```python
from build123d import *

# Parameters (mm, degrees)
SKETCH021_W     = 28
SKETCH021_H     = 45
SKETCH021_R     = 1.5
PAD010_DEPTH    = 6
SKETCH022_W     = 7
SKETCH022_H     = 45
SKETCH022_R     = 1.5
SKETCH022_W_2   = 6
SKETCH022_H_2   = 10
SKETCH022_H_3   = 6
PAD011_DEPTH    = 8
SKETCH032_R     = 3.5
POCKET010_DEPTH = 3
POCKET011_DEPTH = 27
SKETCH034_R     = 1.5
POCKET012_DEPTH = 19
SKETCH035_R     = 5
PAD012_DEPTH    = 11
SKETCH036_R     = 5
PAD013_DEPTH    = 11
SKETCH037_R     = 1.5
POCKET013_DEPTH = 20
SKETCH038_R     = 1.5
POCKET014_DEPTH = 20
CHAMFER005_SIZE = 2
CHAMFER006_SIZE = 2
CHAMFER007_SIZE = 2
SKETCH039_W     = 9
SKETCH039_H     = 2
PAD014_DEPTH    = 8
SKETCH040_W     = 8
SKETCH040_H     = 2
PAD015_DEPTH    = 8
CHAMFER008_SIZE = 6
SKETCH041_W     = 6
SKETCH041_H     = 2.3
POCKET015_DEPTH = 6
CHAMFER012_SIZE = 2
PAD017_DEPTH    = 1
SKETCH047_W     = 2.3
SKETCH047_H     = 6
POCKET018_DEPTH = 9


with BuildPart() as part:
    # Sketch021 → Pad010 (new body)
    with BuildSketch(Plane.XZ):
        with Locations((14, 22.5)):
            Rectangle(SKETCH021_W, SKETCH021_H)
        with Locations((4, 32.5)):
            Circle(SKETCH021_R, mode=Mode.SUBTRACT)
        with Locations((24, 32.5)):
            Circle(SKETCH021_R, mode=Mode.SUBTRACT)
        with Locations((4, 12.5)):
            Circle(SKETCH021_R, mode=Mode.SUBTRACT)
        with Locations((24, 12.5)):
            Circle(SKETCH021_R, mode=Mode.SUBTRACT)
    extrude(amount=PAD010_DEPTH)

    # Sketch022 (on Face9 of Pad010) → Pad011 (join)
    with BuildSketch(Plane(origin=(0, 0, 0), x_dir=(1, 0, 0), z_dir=(0, 1, 0))):
        with Locations((3.5, -22.5)):
            Rectangle(SKETCH022_W, SKETCH022_H)
        with Locations((4, -12.5)):
            Circle(SKETCH022_R, mode=Mode.SUBTRACT)
        with Locations((4, -32.5)):
            Circle(SKETCH022_R, mode=Mode.SUBTRACT)
        with Locations((24.5, -22.5)):
            Rectangle(SKETCH022_W, SKETCH022_H)
        with Locations((24, -12.5)):
            Circle(SKETCH022_R, mode=Mode.SUBTRACT)
        with Locations((24, -32.5)):
            Circle(SKETCH022_R, mode=Mode.SUBTRACT)
        with Locations((15.5, -5)):
            Rectangle(SKETCH022_W_2, SKETCH022_H_2)
        with Locations((15.5, -15)):
            Rectangle(SKETCH022_W_2, SKETCH022_H_3)
    extrude(amount=PAD011_DEPTH)

    # Sketch032 → Pocket010 (cut)
    with BuildSketch(Plane(origin=(0, 8, 0), x_dir=(1, 0, 0), z_dir=(0, 1, 0))):
        with Locations((4, -12.5)):
            Circle(SKETCH032_R)
        with Locations((4, -32.5)):
            Circle(SKETCH032_R)
        with Locations((24, -32.5)):
            Circle(SKETCH032_R)
        with Locations((24, -12.5)):
            Circle(SKETCH032_R)
    extrude(amount=-POCKET010_DEPTH, mode=Mode.SUBTRACT)

    # Sketch033 (on Face4 of Pocket010) → Pocket011 (cut)
    with BuildSketch(Plane(origin=(0, 0, 45), x_dir=(-1, 0, 0), z_dir=(0, 0, 1))):
        Polygon((-22, 6), (-8, 6), (-10, 0), (-21, 0), align=None)
    extrude(amount=-POCKET011_DEPTH, mode=Mode.SUBTRACT)

    # Sketch034 (on Face5 of Pocket011) → Pocket012 (cut)
    with BuildSketch(Plane(origin=(0, 0, 18), x_dir=(-1, 0, 0), z_dir=(0, 0, 1))):
        with Locations((-15.5, 3)):
            Circle(SKETCH034_R)
    extrude(amount=-POCKET012_DEPTH, mode=Mode.SUBTRACT)

    # Sketch035 (on Face14 of Pocket012) → Pad012 (join)
    with BuildSketch(Plane(origin=(0, 0, 0), x_dir=(0, 0, -1), z_dir=(-1, 0, 0))):
        with Locations((-5, -3)):
            Circle(SKETCH035_R)
    extrude(amount=PAD012_DEPTH)

    # Sketch036 (on Face21 of Pocket012) → Pad013 (join)
    with BuildSketch(Plane(origin=(28, 0, 0), x_dir=(0, 0, 1), z_dir=(1, 0, 0))):
        with Locations((5, -3)):
            Circle(SKETCH036_R)
    extrude(amount=PAD013_DEPTH)

    # Sketch037 (on Face35 of Pad013) → Pocket013 (cut)
    with BuildSketch(Plane(origin=(-11, 0, 0), x_dir=(0, 0, -1), z_dir=(-1, 0, 0))):
        with Locations((-5, -3)):
            Circle(SKETCH037_R)
    extrude(amount=-POCKET013_DEPTH, mode=Mode.SUBTRACT)

    # Sketch038 (on Face52 of Pocket013) → Pocket014 (cut)
    with BuildSketch(Plane(origin=(39, 0, 0), x_dir=(0, 0, 1), z_dir=(1, 0, 0))):
        with Locations((5, -3)):
            Circle(SKETCH038_R)
    extrude(amount=-POCKET014_DEPTH, mode=Mode.SUBTRACT)

    # Chamfer005
    chamfer005_edges = [part.edges().sort_by_distance(p)[0] for p in [
        (39, 3, 0),
        (-11, 3, 10),
    ]]
    chamfer(chamfer005_edges, length=CHAMFER005_SIZE)

    # Chamfer006
    chamfer006_edges = [part.edges().sort_by_distance(p)[0] for p in [
        (37, 3, 0),
        (-9, 3, 10),
    ]]
    chamfer(chamfer006_edges, length=CHAMFER006_SIZE)

    # Chamfer007
    chamfer007_edges = [part.edges().sort_by_distance(p)[0] for p in [
        (35, 3, 2.2e-05),
        (-7, 3, 9.999978),
    ]]
    chamfer(chamfer007_edges, length=CHAMFER007_SIZE)

    # Sketch039 (on Face4 of Chamfer007) → Pad014 (join)
    with BuildSketch(Plane(origin=(0, 0, 0), x_dir=(0, 0, -1), z_dir=(-1, 0, 0))):
        with Locations((-12.5, -3)):
            Rectangle(SKETCH039_W, SKETCH039_H)
    extrude(amount=PAD014_DEPTH)

    # Sketch040 (on Face48 of Pad014) → Pad015 (join)
    with BuildSketch(Plane(origin=(28, 0, 0), x_dir=(0, 0, 1), z_dir=(1, 0, 0))):
        with Locations((12, -3)):
            Rectangle(SKETCH040_W, SKETCH040_H)
    extrude(amount=PAD015_DEPTH)

    # Chamfer008
    chamfer008_edges = [part.edges().sort_by_distance(p)[0] for p in [
        (-8, 3, 17),
        (36, 3, 16),
    ]]
    chamfer(chamfer008_edges, length=CHAMFER008_SIZE)

    # Sketch041 (on Face17 of Chamfer008) → Pocket015 (cut)
    with BuildSketch(Plane.XZ.offset(6)):
        with Locations((15.5, 13.85)):
            Rectangle(SKETCH041_W, SKETCH041_H)
    extrude(amount=-POCKET015_DEPTH, mode=Mode.SUBTRACT)

    # Chamfer012
    chamfer012_edges = [part.edges().sort_by_distance(p)[0] for p in [
        (18.5, 4, 10),
    ]]
    chamfer(chamfer012_edges, length=CHAMFER012_SIZE)

    # Sketch045 (on Face18 of Chamfer012) → Pad017 (join)
    with BuildSketch(Plane(origin=(0, 8, 0), x_dir=(1, 0, 0), z_dir=(0, 1, 0))):
        Polygon((12.5, 0), (21, 0), (21, -10.697224), (18.5, -12), (18.5, -18), (12.5, -18), align=None)
    extrude(amount=-PAD017_DEPTH)

    # Sketch047 (on Face25 of Pad017) → Pocket018 (cut)
    with BuildSketch(Plane(origin=(0, 8, 0), x_dir=(1, 0, 0), z_dir=(0, 1, 0))):
        with Locations((3.15, -5)):
            Rectangle(SKETCH047_W, SKETCH047_H)
        with Locations((24.85, -5)):
            Rectangle(SKETCH047_W, SKETCH047_H)
    extrude(amount=-POCKET018_DEPTH, mode=Mode.SUBTRACT)


with BuildPart() as part_1:
    # Body007 placement: moved
    add(part.part.moved(Location((-14, 27.5, 3))))


solid = part_1.part
```
Check sheet for the modelled part. Datum: model origin and axes. Units: mm. A direction names the side the tool comes from. Round coordinates to 2 decimals unless told otherwise and drop trailing zeros. Loops run counter-clockwise (first coordinate to the right, second up) from the corner with the lowest first, then second, coordinate; pieces in that order, holes last. Notation, with made-up numbers: (57, 67) -> (95, 67) arc R36 cw to (95, 104) -> close; hole circle Ø8 at (-35, -27.5). An arc over 180 degrees is marked (long way). Answer in a Markdown table with one row per item.
Q1. Sectioned sample at C-C on z = 35.5. Enter the section's corners in (x, y), then the cut area to 3 significant figures.
Data:
| item | result |
|---|---|
| outline | (-14, 21.5) -> (-11.5, 21.5) -> (-11.5, 32.5) -> (-13.5, 32.5) -> (-13.5, 35.5) -> (-14, 35.5) -> close; (-8.5, 21.5) -> (-6, 21.5) -> (-4, 27.5) -> (-7, 27.5) -> (-7, 32.5) -> (-8.5, 32.5) -> close; (7, 27.5) -> (8, 21.5) -> (8.5, 21.5) -> (8.5, 32.5) -> (7, 32.5) -> close; (11.5, 21.5) -> (14, 21.5) -> (14, 35.5) -> (13.5, 35.5) -> (13.5, 32.5) -> (11.5, 32.5) -> close |
| area | 100 mm^2 |
Q2. Go/stop test with flat-tipped pins: P1, Ø5, axis at x = 1.5, y = 24.5, coming from the +Z side; P2, Ø5, axis at x = -9, z = 35.5, coming from the +Y side; P3, Ø2.5, axis at y = 30.5, z = 8, coming from the -X side; P4, Ø8, axis at x = 10, z = 15.5, coming from the +Y side. Record where each tip stops, or that it passes through.
Data:
| item | result |
|---|---|
| P1 | stops at z = 21 |
| P2 | stops at y = 32.5 |
| P3 | stops at x = -1.5 |
| P4 | stops at y = 35.5 |
Q3. Thickness scan on L1, parallel to Z at x = 10, y = 27.5; L2, parallel to Z at x = -10, y = 34.3; L3, parallel to Z at x = -10, y = 25.5. Record the ranges inside material, lowest first.
Data:
| item | result |
|---|---|
| L1 | z = 3 to 5, 11 to 14, 17 to 34, 37 to 48 |
| L2 | z = 3 to 5, 11 to 12, 19 to 32, 39 to 48 |
| L3 | z = 3 to 14, 17 to 34, 37 to 48 |
Q4. Sectioned sample at B-B on x = 1.5. Enter the section's corners in (y, z).
Data:
| item | result |
|---|---|
| outline | (21.5, 3) -> (23, 3) -> (23, 15.7) -> (21.5, 15.7) -> close; (21.5, 18) -> (23, 18) -> (23, 21) -> (21.5, 21) -> close; (26, 3) -> (35.5, 3) -> (35.5, 21) -> (26, 21) -> (26, 18) -> (27.5, 18) -> (27.5, 15.7) -> (26, 15.7) -> close; hole (27.5, 13) -> (34.5, 13) -> (34.5, 15) -> (27.5, 15) -> close |
Q5. Release check for a two-part mould opening along Y. For faces 1 (the face through (-12, 32.5, 15)), 2 (the face through (0, 31, 13)), 3 (the face through (0, 28, 3)) record: released by +Y, released by -Y, zero draft, split by the parting line, or undercut.
Data:
| item | result |
|---|---|
| face 1 | released by +Y |
| face 2 | undercut |
| face 3 | zero draft |
Q6. Set-up check for faces 4 (the face through (16.465, 30.294, 3.004)), 5 (the face through (5, 34.5, 10)), 6 (the face through (17, 31.5, 16)), 7 (the face through (0, 23, 18)), 8 (the face through (-13.5, 34, 35.4)): record each of +Z, -Z, +X, -X, +Y, -Y from which the full face is reachable in a straight line by a thin tool's end or side.
Data:
| item | result |
|---|---|
| face 4 | +X |
| face 5 | none |
| face 6 | +Z, +X, +Y |
| face 7 | -Y |
| face 8 | +Y |
Q7. Sectioned sample at D-D on x = 18. Enter the section's corners in (y, z).
Data:
| item | result |
|---|---|
| outline | (29.5, 12.9) arc R5 ccw (long way) to (31.5, 12.9) -> (31.5, 17) -> (29.5, 17) -> close; hole circle Ø3 at (30.5, 8) |
Q8. Sectioned sample at A-A on z = 22.5. Enter the section's corners in (x, y), then the cut area to 3 significant figures.
Data:
| item | result |
|---|---|
| outline | (-14, 21.5) -> (-6, 21.5) -> (-4, 27.5) -> (-7, 27.5) -> (-7, 35.5) -> (-14, 35.5) -> close; (7, 27.5) -> (8, 21.5) -> (14, 21.5) -> (14, 35.5) -> (7, 35.5) -> close |
| area | 205 mm^2 |
